```python
from build123d import *

# Parameters (mm, degrees)
SHELL1_T         = -8.466666667
EXTRUSION3_DEPTH = 8.466666667
EXTRUSION4_DEPTH = 8.466666667
EXTRUSION5_DEPTH = 8.466666667
EXTRUSION6_DEPTH = 8.466666667


with BuildPart() as part:
    # Extrusion2: read off the stored shape, not the designer's step
    # Extrusion2: loft between two sections, ruled curve by curve
    extrusion2_from = [
        Edge.make_line((-482.6, -222.25, 2.54), (482.6, -222.25, 2.54)),
        Edge.make_line((-482.6, 222.25, 2.54), (-482.6, -222.25, 2.54)),
        Edge.make_line((482.6, 222.25, 2.54), (-482.6, 222.25, 2.54)),
        Edge.make_line((482.6, -222.25, 2.54), (482.6, 222.25, 2.54)),
    ]
    extrusion2_to = [
        Edge.make_line((-19.05, -9.525, 1018.54), (19.05, -9.525, 1018.54)),
        Edge.make_line((-19.05, 9.525, 1018.54), (-19.05, -9.525, 1018.54)),
        Edge.make_line((19.05, 9.525, 1018.54), (-19.05, 9.525, 1018.54)),
        Edge.make_line((19.05, -9.525, 1018.54), (19.05, 9.525, 1018.54)),
    ]
    extrusion2 = Solid(Shell([*[Face.make_surface_from_curves(extrusion2_from[k], extrusion2_to[k]) for k in range(4)], Face(Wire(extrusion2_from)), Face(Wire(extrusion2_to))]))
    add(extrusion2)

    # Shell1
    shell1_openings = [part.faces().sort_by_distance(p)[0] for p in [
        (0, 0, 2.54),
    ]]
    offset(amount=SHELL1_T, openings=shell1_openings, kind=Kind.INTERSECTION)

    # Sketch2 → Extrusion3 (cut)
    with BuildSketch(Plane(origin=(400.408264089, 0, 182.68627049), x_dir=(0.4150877539122262, 0, -0.9097813784377559), z_dir=(0.909781378437756, 0, 0.41508775391222624))):
        Polygon((-917.157013109, 1.207881), (-917.157013109, -1.207881), (198.010505337, -213.631096694), (198.010505337, 213.631096694), align=None)
    extrude(amount=-EXTRUSION3_DEPTH, mode=Mode.SUBTRACT)

    # Sketch3 → Extrusion4 (cut)
    with BuildSketch(Plane(origin=(-400.408264089, 0, 182.68627049), x_dir=(0.4150877539122262, 0, 0.9097813784377559), z_dir=(-0.909781378437756, 0, 0.41508775391222624))):
        Polygon((917.157013109, -1.207881), (917.157013109, 1.207881), (-198.010505337, 213.631096694), (-198.010505337, -213.631096694), align=None)
    extrude(amount=-EXTRUSION4_DEPTH, mode=Mode.SUBTRACT)

    # Sketch4 → Extrusion5 (cut)
    with BuildSketch(Plane(origin=(0, 213.425680846, 44.686001927), x_dir=(-1, 0, 0), z_dir=(0, 0.9787763596240335, 0.204931300296282))):
        Polygon((-11.319163518, 991.518568451), (-473.327465959, -43.059889537), (473.327465959, -43.059889537), (11.319163518, 991.518568451), align=None)
    extrude(amount=-EXTRUSION5_DEPTH, mode=Mode.SUBTRACT)

    # Sketch5 → Extrusion6 (cut)
    with BuildSketch(Plane(origin=(0, -213.425680846, 44.686001927), x_dir=(1, 0, 0), z_dir=(0, -0.9787763596240335, 0.204931300296282))):
        Polygon((-11.319163518, 991.518568451), (-473.327465959, -43.059889537), (473.327465959, -43.059889537), (11.319163518, 991.518568451), align=None)
    extrude(amount=-EXTRUSION6_DEPTH, mode=Mode.SUBTRACT)


solid = part.part
```
Geometry: final body of the model. Coordinates: model frame, mm. A direction names the side the tool comes from. Coordinates: 2 decimals unless noted, no trailing zeros. Answer in a Markdown table with one row per item.
Item 1: Contact query for flat-ended pins moving along their axis: P1, Ø4, axis at y = -156, z = 294.5, coming from the +X side; P2, Ø1.6, axis at x = 3, y = -1, coming from the -Z side. Output: stop coordinate, or through.
Return value:
| item | result |
|---|---|
| P1 | stops at x = 350.31 |
| P2 | stops at z = 1010.07 |
Item 2: Draft query along Y for faces 1 (the flat face through (239.09, 110.67, 515.08)), 2 (the flat face through (-244.116, 105.933, 515.189)), 3 (the flat face through (245.557, -113.64, 500.907)). Return one class per face: released by +Y, released by -Y, zero draft, split by the parting line, or undercut.
Return value:
| item | result |
|---|---|
| face 1 | released by +Y |
| face 2 | undercut |
| face 3 | released by -Y |
Item 3: Section A-A on z = 876. State how many separate pieces and enclosed holes the cut face has, plus the area to 3 significant figures.
Return value:
| item | result |
|---|---|
| separate pieces | 4 |
| enclosed holes | 0 |
| area | 347 mm² |
Item 4: Access query for faces 4 (the flat face through (-250.597, -108.906, 500.985)), 5 (the flat face through (250.597, 108.906, 500.985)). Directions: +Z, -Z, +X, -X, +Y, -Y. A direction counts if a zero-diameter tool reaches every point of the face in a straight line with its end or side. Return the directions, or none.
Return value:
| item | result |
|---|---|
| face 4 | -Z, -X |
| face 5 | -Z, +X |
